Verification items for the finished model (mm, model axes). Face numbers are marked on the shaded views. Coordinates: 2 decimals unless noted, no trailing zeros. Loops run counter-clockwise (first coordinate to the right, second up) from the corner with the lowest first, then second, coordinate; pieces in that order, holes last. Notation, with made-up numbers: (21.25, 60) -> (70.25, 60) arc R22 cw to (70.25, 90) -> close; hole circle Ø10 at (24.25, 1.25). An arc over 180 degrees is marked (long way). Write item = value, one per line.
```python
from build123d import *

# Parameters (mm, degrees)
SKETCH1_R               = 8.382
BOSS_EXTRUDE1_DEPTH     = 1.27
SKETCH2_R               = 5.588
BOSS_EXTRUDE2_DEPTH     = 7.112
SKETCH3_R               = 8.382
BOSS_EXTRUDE3_DEPTH     = 1.27
SKETCH4_R               = 2.54
CUT_EXTRUDE1_DEPTH      = 1
CUT_EXTRUDE1_DEPTH_BACK = 10.652
CHAMFER1_SIZE           = 0.508


with BuildPart() as part:
    # Sketch1 → Boss-Extrude1 (new body)
    with BuildSketch(Plane(origin=(0, 0, 0), x_dir=(1, 0, 0), z_dir=(0, 1, 0))):
        Circle(SKETCH1_R)
    extrude(amount=-BOSS_EXTRUDE1_DEPTH)

    # Sketch2 → Boss-Extrude2 (add)
    with BuildSketch(Plane(origin=(0, 0, 0), x_dir=(1, 0, 0), z_dir=(0, 1, 0))):
        with BuildLine():
            ThreePointArc((-4.121307864, 3.77366738), (-4.666752119, 3.721610627), (-4.596130935, 3.178258081))
            ThreePointArc((-4.596130935, 3.178258081), (-4.368874324, 3.484061013), (-4.121307864, 3.77366738))
        make_face()
        with BuildLine():
            ThreePointArc((-4.857698061, 2.761976385), (-5.377883173, 2.589852039), (-5.188125293, 2.075837167))
            ThreePointArc((-5.188125293, 2.075837167), (-5.034614034, 2.424542334), (-4.857698061, 2.761976385))
        make_face()
        with BuildLine():
            ThreePointArc((-5.350502993, 1.611788361), (-5.819344708, 1.328227455), (-5.519965385, 0.86932511))
            ThreePointArc((-5.519965385, 0.86932511), (-5.447897173, 1.243446979), (-5.350502993, 1.611788361))
        make_face()
        with BuildLine():
            ThreePointArc((-5.575011364, 0.380778538), (-5.969, 0), (-5.575011364, -0.380778538))
            ThreePointArc((-5.575011364, -0.380778538), (-5.588, 0), (-5.575011364, 0.380778538))
        make_face()
        with BuildLine():
            ThreePointArc((-5.350502993, -1.611788361), (-5.447897173, -1.243446979), (-5.519965385, -0.86932511))
            ThreePointArc((-5.519965385, -0.86932511), (-5.819344708, -1.328227455), (-5.350502993, -1.611788361))
        make_face()
        with BuildLine():
            ThreePointArc((-4.857698061, -2.761976385), (-5.034614034, -2.424542334), (-5.188125293, -2.075837167))
            ThreePointArc((-5.188125293, -2.075837167), (-5.377883173, -2.589852039), (-4.857698061, -2.761976385))
        make_face()
        with BuildLine():
            ThreePointArc((-4.121307864, -3.77366738), (-4.368874324, -3.484061013), (-4.596130935, -3.178258081))
            ThreePointArc((-4.596130935, -3.178258081), (-4.666752119, -3.721610627), (-4.121307864, -3.77366738))
        make_face()
        with BuildLine():
            ThreePointArc((-2.075837167, -5.188125293), (-2.424542334, -5.034614034), (-2.761976385, -4.857698061))
            ThreePointArc((-2.761976385, -4.857698061), (-2.589852039, -5.377883173), (-2.075837167, -5.188125293))
        make_face()
        with BuildLine():
            ThreePointArc((-0.86932511, -5.519965385), (-1.243446979, -5.447897173), (-1.611788361, -5.350502993))
            ThreePointArc((-1.611788361, -5.350502993), (-1.328227455, -5.819344708), (-0.86932511, -5.519965385))
        make_face()
        with BuildLine():
            ThreePointArc((2.761976385, -4.857698061), (2.424542334, -5.034614034), (2.075837167, -5.188125293))
            ThreePointArc((2.075837167, -5.188125293), (2.589852039, -5.377883173), (2.761976385, -4.857698061))
        make_face()
        with BuildLine():
            ThreePointArc((3.77366738, -4.121307864), (3.484061013, -4.368874324), (3.178258081, -4.596130935))
            ThreePointArc((3.178258081, -4.596130935), (3.721610627, -4.666752119), (3.77366738, -4.121307864))
        make_face()
        with BuildLine():
            ThreePointArc((4.596130935, -3.178258081), (4.368874324, -3.484061013), (4.121307864, -3.77366738))
            ThreePointArc((4.121307864, -3.77366738), (4.666752119, -3.721610627), (4.596130935, -3.178258081))
        make_face()
        with BuildLine():
            ThreePointArc((5.188125293, -2.075837167), (5.034614034, -2.424542334), (4.857698061, -2.761976385))
            ThreePointArc((4.857698061, -2.761976385), (5.377883173, -2.589852039), (5.188125293, -2.075837167))
        make_face()
        with BuildLine():
            ThreePointArc((5.588, 0), (5.584751897, -0.1905), (5.575011364, -0.380778538))
            ThreePointArc((5.575011364, -0.380778538), (5.969, 0), (5.575011364, 0.380778538))
            ThreePointArc((5.575011364, 0.380778538), (5.584751897, 0.1905), (5.588, 0))
        make_face()
        with BuildLine():
            ThreePointArc((5.519965385, 0.86932511), (5.819344708, 1.328227455), (5.350502993, 1.611788361))
            ThreePointArc((5.350502993, 1.611788361), (5.447897173, 1.243446979), (5.519965385, 0.86932511))
        make_face()
        with BuildLine():
            ThreePointArc((5.188125293, 2.075837167), (5.377883173, 2.589852039), (4.857698061, 2.761976385))
            ThreePointArc((4.857698061, 2.761976385), (5.034614034, 2.424542334), (5.188125293, 2.075837167))
        make_face()
        with BuildLine():
            ThreePointArc((4.596130935, 3.178258081), (4.666752119, 3.721610627), (4.121307864, 3.77366738))
            ThreePointArc((4.121307864, 3.77366738), (4.368874324, 3.484061013), (4.596130935, 3.178258081))
        make_face()
        with BuildLine():
            ThreePointArc((3.77366738, 4.121307864), (3.721610627, 4.666752119), (3.178258081, 4.596130935))
            ThreePointArc((3.178258081, 4.596130935), (3.484061013, 4.368874324), (3.77366738, 4.121307864))
        make_face()
        with BuildLine():
            ThreePointArc((2.761976385, 4.857698061), (2.589852039, 5.377883173), (2.075837167, 5.188125293))
            ThreePointArc((2.075837167, 5.188125293), (2.424542334, 5.034614034), (2.761976385, 4.857698061))
        make_face()
        with BuildLine():
            ThreePointArc((1.611788361, 5.350502993), (1.328227455, 5.819344708), (0.86932511, 5.519965385))
            ThreePointArc((0.86932511, 5.519965385), (1.243446979, 5.447897173), (1.611788361, 5.350502993))
        make_face()
        with BuildLine():
            ThreePointArc((0.380778538, 5.575011364), (0, 5.969), (-0.380778538, 5.575011364))
            ThreePointArc((-0.380778538, 5.575011364), (0, 5.588), (0.380778538, 5.575011364))
        make_face()
        with BuildLine():
            ThreePointArc((-0.86932511, 5.519965385), (-1.328227455, 5.819344708), (-1.611788361, 5.350502993))
            ThreePointArc((-1.611788361, 5.350502993), (-1.243446979, 5.447897173), (-0.86932511, 5.519965385))
        make_face()
        with BuildLine():
            ThreePointArc((-2.075837167, 5.188125293), (-2.589852039, 5.377883173), (-2.761976385, 4.857698061))
            ThreePointArc((-2.761976385, 4.857698061), (-2.424542334, 5.034614034), (-2.075837167, 5.188125293))
        make_face()
        with BuildLine():
            ThreePointArc((-3.178258081, 4.596130935), (-3.721610627, 4.666752119), (-3.77366738, 4.121307864))
            ThreePointArc((-3.77366738, 4.121307864), (-3.484061013, 4.368874324), (-3.178258081, 4.596130935))
        make_face()
        with BuildLine():
            ThreePointArc((-3.178258081, -4.596130935), (-3.484061013, -4.368874324), (-3.77366738, -4.121307864))
            ThreePointArc((-3.77366738, -4.121307864), (-3.721610627, -4.666752119), (-3.178258081, -4.596130935))
        make_face()
        with BuildLine():
            ThreePointArc((0.380778538, -5.575011364), (0, -5.588), (-0.380778538, -5.575011364))
            ThreePointArc((-0.380778538, -5.575011364), (0, -5.969), (0.380778538, -5.575011364))
        make_face()
        with BuildLine():
            ThreePointArc((1.611788361, -5.350502993), (1.243446979, -5.447897173), (0.86932511, -5.519965385))
            ThreePointArc((0.86932511, -5.519965385), (1.328227455, -5.819344708), (1.611788361, -5.350502993))
        make_face()
        with BuildLine():
            ThreePointArc((5.519965385, -0.86932511), (5.447897173, -1.243446979), (5.350502993, -1.611788361))
            ThreePointArc((5.350502993, -1.611788361), (5.819344708, -1.328227455), (5.519965385, -0.86932511))
        make_face()
        Circle(SKETCH2_R)
    extrude(amount=BOSS_EXTRUDE2_DEPTH)

    # Sketch3 → Boss-Extrude3 (add)
    with BuildSketch(Plane(origin=(0, 7.112, 0), x_dir=(1, 0, 0), z_dir=(0, 1, 0))):
        Circle(SKETCH3_R)
    extrude(amount=BOSS_EXTRUDE3_DEPTH)

    # Sketch4 → Cut-Extrude1 (cut, two sides)
    with BuildSketch(Plane.XZ.offset(1.27)) as cut_extrude1_sk:
        Circle(SKETCH4_R)
    extrude(amount=CUT_EXTRUDE1_DEPTH, mode=Mode.SUBTRACT)
    extrude(cut_extrude1_sk.sketch, amount=-CUT_EXTRUDE1_DEPTH_BACK, mode=Mode.SUBTRACT)

    # Chamfer1
    chamfer1_edges = [part.edges().sort_by_distance(p)[0] for p in [
        (-2.54, 8.382, 0),
        (-2.54, -1.27, 0),
    ]]
    chamfer(chamfer1_edges, length=CHAMFER1_SIZE)


solid = part.part
```
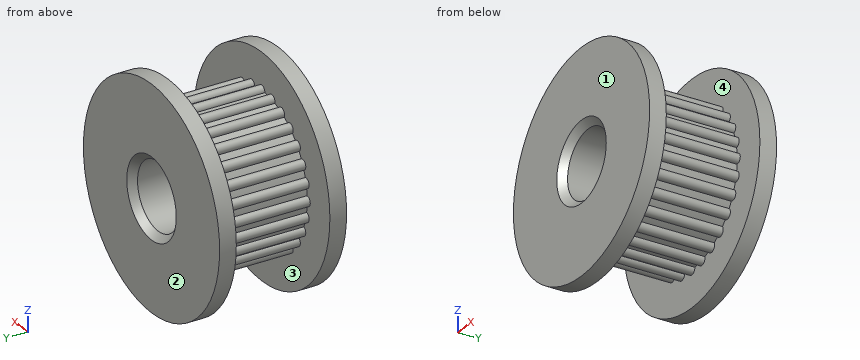
1) Sectioned sample at D-D, the plane z = -7.25. Record the cut outline in (x, y).
Ans:
outline = (-4.21, -1.27) -> (4.21, -1.27) -> (4.21, 0) -> (-4.21, 0) -> close; (-4.21, 7.11) -> (4.21, 7.11) -> (4.21, 8.38) -> (-4.21, 8.38) -> close
2) Depth check by flat-ended pin: pin 1 Ø1.5 at (y, z) = (2.5, -3) entering from +X; pin 2 Ø5 at (x, y) = (3.5, 1) entering from +Z; pin 3 Ø1 at (x, y) = (3.5, 1) entering from -Z. Enter the tip coordinate at first touch or a pass-through.
Ans:
pin_1 = 5.42
pin_2 = 8.29
pin_3 = -4.75
3) Material ranges on line 1 (Z direction, x = 0, y = 4.25); line 2 (Y direction, x = 3.25, z = -7); line 3 (Z direction, x = -3.5, y = 4.5), recorded low to high.
Ans:
line_1 = -5.97 to -2.54, 2.54 to 5.97
line_2 = -1.27 to 0, 7.11 to 8.38
line_3 = -4.75 to 4.75
4) Sectioned sample at C-C, the plane y = 7.5. Record the cut outline in (x, z).
Ans:
outline = circle Ø16.76 at (0, 0); hole circle Ø5.08 at (0, 0)
5) Sectioned sample at B-B, the plane z = 0. Record the cut outline in (x, y), plus the area to 3 significant figures.
Ans:
outline = (-8.38, -1.27) -> (-3.05, -1.27) -> (-2.54, -0.76) -> (-2.54, 7.87) -> (-3.05, 8.38) -> (-8.38, 8.38) -> (-8.38, 7.11) -> (-5.97, 7.11) -> (-5.97, 0) -> (-8.38, 0) -> close; (2.54, -0.76) -> (3.05, -1.27) -> (8.38, -1.27) -> (8.38, 0) -> (5.97, 0) -> (5.97, 7.11) -> (8.38, 7.11) -> (8.38, 8.38) -> (3.05, 8.38) -> (2.54, 7.87) -> close
area = 77.9 mm2
6) Sectioned sample at A-A, the plane x = 0. Record the cut outline in (y, z), plus the area to 3 significant figures.
Ans:
outline = (-1.27, -8.38) -> (0, -8.38) -> (0, -5.97) -> (7.11, -5.97) -> (7.11, -8.38) -> (8.38, -8.38) -> (8.38, -3.05) -> (7.87, -2.54) -> (-0.76, -2.54) -> (-1.27, -3.05) -> close; (-1.27, 3.05) -> (-0.76, 2.54) -> (7.87, 2.54) -> (8.38, 3.05) -> (8.38, 8.38) -> (7.11, 8.38) -> (7.11, 5.97) -> (0, 5.97) -> (0, 8.38) -> (-1.27, 8.38) -> close
area = 77.9 mm2
7) Release check for a two-part mould opening along Y. For the marked faces 1, 2, 3 and 4 record: pulls with the +Y half, pulls with the -Y half, needs draft (parallel to the pull), parting line crosses it, or undercut.
Ans:
face_1 = pulls with the -Y half
face_2 = pulls with the +Y half
face_3 = undercut
face_4 = undercut
